Model file for the job. Use its own axes, mm. Face numbers are marked on the shaded views. A direction names the side the tool comes from. Give positions to 0.01 mm unless a question says otherwise; leave off trailing zeros. Write each loop counter-clockwise with the first axis right and the second up, starting at its lowest first coordinate (ties: lowest second). Pieces come first, ordered by that corner, then holes.
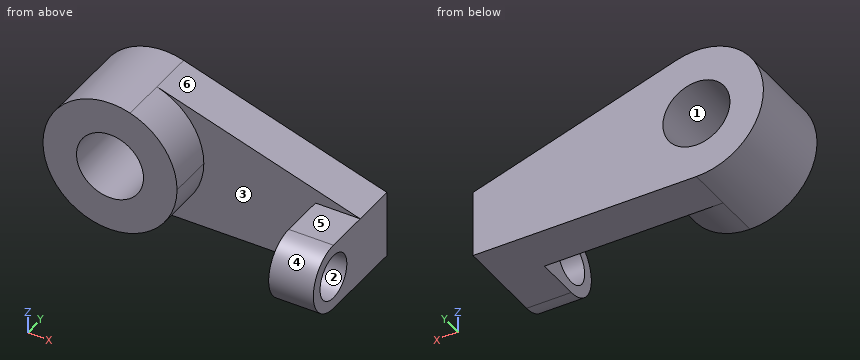
```python
from build123d import *

# Parameters (mm, degrees)
F0_R     = 7.5
F1_DEPTH = 10
F2_DEPTH = 20
F3_R     = 5
F4_DEPTH = 10


with BuildPart() as f1:
    # F0 (on Front) → F1 (new body)
    with BuildSketch(Plane.XZ):
        with BuildLine():
            ThreePointArc((0, -15), (10.606602, -10.606602), (15, 0))
            ThreePointArc((15, 0), (12.093387, 8.87412), (4.5, 14.309088))
            ThreePointArc((4.5, 14.309088), (-14.826266, 2.276365), (0, -15))
        make_face()
        Circle(F0_R, mode=Mode.SUBTRACT)
        with BuildLine():
            ThreePointArc((4.5, 14.309088), (12.093387, 8.87412), (15, 0))
            ThreePointArc((15, 0), (10.606602, -10.606602), (0, -15))
            Line((0, -15), (50, -15))
            Line((50, -15), (50, 0))
            Line((50, 0), (4.5, 14.309088))
        make_face()
    extrude(amount=F1_DEPTH)

    # F0 (on Front) → F2 (join)
    with BuildSketch(Plane.XZ):
        with BuildLine():
            ThreePointArc((0, -15), (10.606602, -10.606602), (15, 0))
            ThreePointArc((15, 0), (12.093387, 8.87412), (4.5, 14.309088))
            ThreePointArc((4.5, 14.309088), (-14.826266, 2.276365), (0, -15))
        make_face()
        Circle(F0_R, mode=Mode.SUBTRACT)
    extrude(amount=F2_DEPTH)

    # F3 (on face) → F4 (join)
    with BuildSketch(Plane.YZ.offset(50)):
        with BuildLine():
            Line((-20, -15), (0, -15))
            Line((0, -15), (0, 0))
            Line((0, 0), (-20, 0))
            ThreePointArc((-20, 0), (-27.5, -7.5), (-20, -15))
        make_face()
        with Locations((-20, -7.5)):
            Circle(F3_R, mode=Mode.SUBTRACT)
    extrude(amount=-F4_DEPTH)


solid = f1.part
```
1. Pin check, flat tips, straight feed: P1, Ø8, axis at y = -7.5, z = 8, coming from the -X side; P2, Ø11.5, axis at y = -20, z = -7.5, coming from the -X side; P3, Ø10, axis at x = 37, y = -13, coming from the +Z side. Stop position of each tip, or through.
Calculated:
P1: stops at x = -14.46
P2: stops at x = -14.9
P3: stops at z = 5.35
2. Slice it at D-D, the plane z = -8.25. Write the cut outline in (x, y).
Calculated:
outline: (-12.53, -20) - (12.53, -20) - (12.53, -10) - (40, -10) - (40, -15.06) - (50, -15.06) - (50, 0) - (-12.53, 0) - close; (40, -27.46) - (50, -27.46) - (50, -24.94) - (40, -24.94) - close
3. Pull direction Z, two halves, no side cores. Call the marked faces 1, 2, 3 and 4: +Z half, -Z half, draft (parallel to the pull), parting line (faces both ways), or undercut.
Calculated:
face 1: undercut
face 2: undercut
face 3: draft
face 4: parting line
4. Which spindle directions (+Z, -Z, +X, -X, +Y, -Y) get a long thin tool onto all of the face, cutting with end or side? Do the marked faces 5 and 6. Say none if no direction does.
Calculated:
face 5: +Z, +X, -Y
face 6: +Z, +X, +Y, -Y
5. Slice it at A-A, the plane y = -12. Write the cut outline in (x, z), and give its area (3 significant figures).
Calculated:
outline: (0, -15) arc R15 ccw to (15, 0) arc R15 ccw to (4.5, 14.31) arc R15 ccw (long way) to start; (40, -15) - (50, -15) - (50, 0) - (40, 0) - close; hole circle Ø15 at (0, 0)
area: 680 mm2
6. Probe probe 1 along Z at (x, y) = (45, -20); probe 2 along X at (y, z) = (-7, -0.25); probe 3 along Z at (x, y) = (0, -12.75). List the from-to ranges inside material, lowest first.
Calculated:
probe 1: z = -15 to -12.5, -2.5 to 0
probe 2: x = -15 to -7.5, 7.5 to 50
probe 3: z = -15 to -7.5, 7.5 to 15
7. Slice it at B-B, the plane z = -4. Write the cut outline in (x, y).
Calculated:
outline: (-14.46, -20) - (-6.34, -20) - (-6.34, 0) - (-14.46, 0) - close; (6.34, -20) - (14.46, -20) - (14.46, -10) - (40, -10) - (40, -16.43) - (50, -16.43) - (50, 0) - (6.34, 0) - close; (40, -26.63) - (50, -26.63) - (50, -23.57) - (40, -23.57) - close
